Build history of the part. All positions in model axes, mm. Give positions to 0.01 mm unless a question says otherwise; leave off trailing zeros. Order: outer loops, then holes, each group sorted by start corner. A loop starts at its lowest first (then second) coordinate and runs counter-clockwise, first axis right, second up. Notation, with made-up numbers: M 16.25,4 L 49.25,4 A30 ccw 49.25,29 Z; hole C 89.25,-9 d2. An arc over 180 degrees is marked long. Use CSV: the item, a comma, the result in double quotes. Start each with the question number.
Item 1: Band-saw the part on A-A on y = 0. Write the cut outline in (x, z).
Item 2: Band-saw the part on C-C on z = -34.5. Write the cut outline in (x, y), plus the area to 3 significant figures.
Item 3: Band-saw the part on D-D on z = -16. Write the cut outline in (x, y).
Item 4: Two-plate mould, pull along X, no slides. Class faces 1 (the conical face through (4.703, 4.312, -22.027)), 2 (the cylindrical face through (3, 0, -21)): pulls with the +X half, pulls with the -X half, needs draft (parallel to the pull), parting line crosses it, or undercut.
Item 5: Pin check, flat tips, straight feed: P1, Ø3, axis at x = 1.5, y = -1, coming from the -Z side; P2, Ø4, axis at y = -2, z = -29, coming from the -X side; P3, Ø10, axis at x = -7.5, z = -27.5, coming from the +Y side; P4, Ø5, axis at x = -5, z = -21.5, coming from the +Y side. Stop position of each tip, or through.
Item 6: Wall check: line 1 along Y through (x, z) = (0, -31); line 2 along Y through (x, z) = (0, -25); line 3 along X through (y, z) = (1.5, -34). Give the ranges that are in metal, low to high.
from build123d import *

# Parameters (mm, degrees)
SKETCH_2_R          = 3
CUT_EXTRUDE_1_DEPTH = 11
SKETCH_3_R          = 3
EXTRUDE_1_DEPTH     = 40
SKETCH_5_R          = 3
CUT_EXTRUDE_2_DEPTH = 40


with BuildPart() as part:
    # 草图1 → 旋转1 (revolve)
    with BuildSketch(Plane.XY):
        with BuildLine():
            Line((4.143240259, -9.101294422), (-4.143240259, 9.101294422))
            ThreePointArc((-4.143240259, 9.101294422), (-9.101294422, -4.143240259), (4.143240259, -9.101294422))
        make_face()
    revolve(axis=Axis((4.143240259, -9.101294422, 0), (-0.414324026, 0.910129442, 0)))

    # 草图2 → 切除-拉伸1 (cut, through all)
    with BuildSketch(Plane.XY):
        Circle(SKETCH_2_R)
    extrude(amount=-CUT_EXTRUDE_1_DEPTH, mode=Mode.SUBTRACT)

    # 草图3 → 凸台-拉伸1 (add)
    with BuildSketch(Plane(origin=(0, 0, 0), x_dir=(-1, 0, 0), z_dir=(0, 0, -1))):
        Circle(SKETCH_3_R)
    extrude(amount=EXTRUDE_1_DEPTH)

    # 草图4 → 旋转2 (revolve)
    with BuildSketch(Plane(origin=(0, 0, 0), x_dir=(1, 0, 0), z_dir=(0, 1, 0))):
        Polygon((-3, 0.512695407), (-9.857091429, 1.684561833), (-3, 41.808335168), align=None)
    revolve(axis=Axis((0, 0, 0), (0, 0, -1)))

    # 草图5 → 切除-拉伸2 (cut)
    with BuildSketch(Plane(origin=(0, 0, -40), x_dir=(-1, 0, 0), z_dir=(0, 0, -1))):
        Circle(SKETCH_5_R)
    extrude(amount=-CUT_EXTRUDE_2_DEPTH, mode=Mode.SUBTRACT)


solid = part.part
Model answer:
1,outline,"M -9.86,-1.68 L -3,-41.81 L -3,0 L 3,0 L 3,-41.81 L 9.86,-1.68 A10 ccw long Z"
2,outline,"C 0,0 d8.5; hole C 0,0 d6"
2,area,"28.4 mm^2"
3,outline,"C 0,0 d14.82; hole C 0,0 d6"
4,face 1,"parting line crosses it"
4,face 2,"undercut"
5,P1,"stops at z = -41.81"
5,P2,"stops at x = -5.4"
5,P3,"stops at y = 5.01"
5,P4,"stops at y = 6.06"
6,line 1,"y = -4.85 to -3, 3 to 4.85"
6,line 2,"y = -5.87 to -3, 3 to 5.87"
6,line 3,"x = -4.07 to -2.6, 2.6 to 4.07"
